Input: part model. Units: mm. Frame: model coordinates. A direction names the side the tool comes from. Round coordinates to 2 decimals unless told otherwise and drop trailing zeros. Loops run counter-clockwise (first coordinate to the right, second up) from the corner with the lowest first, then second, coordinate; pieces in that order, holes last. Notation, with made-up numbers: M -30.75,82 L -15.75,82 A24 cw -15.75,93 Z; hole C -25.5,57.25 d5. An arc over 180 degrees is marked long. Return JSON: item names as keys, results as strings. Group by question number.
1) Mould query, pull axis X, two halves, no side actions, for faces 1 (the face through (-29, 8, -32)), 2 (the face through (33, 8, 36)), 3 (the face through (7, 5, -1)). Classes: +X half, -X half, draft (parallel to the pull), parting line (faces both ways), or undercut.
2) Access query for faces 4 (the face through (28, 10, -38)), 5 (the face through (35, 2, 1)), 6 (the face through (29, 8, -32)), 7 (the face through (25, 8, -36)), 8 (the face through (4.75, 3, 0)). Directions: +Z, -Z, +X, -X, +Y, -Y. A direction counts if a zero-diameter tool reaches every point of the face in a straight line with its end or side. Return the directions, or none.
3) Contact query for flat-ended pins moving along their axis: P1, Ø2, axis at y = 7.5, z = -36, coming from the -X side; P2, Ø3, axis at x = 29, z = -36, coming from the -Y side; P3, Ø3, axis at y = 8.5, z = -38, coming from the +X side; P4, Ø4, axis at x = 21.5, z = -17.5, coming from the +Y side. Output: stop coordinate, or through.
4) Section A-A (z = 2). Output: boundary loops of the cut face in (x, y), plus the area to 4 significant figures.
5) Section B-B (y = 7). Output: boundary loops of the cut face in (x, z), plus the area to 3 significant figures.
6) Section C-C (z = 36). Output: boundary loops of the cut face in (x, y).
7) Material intervals for line 1 (X direction, y = 6.5, z = -36); line 2 (X direction, y = 3, z = 36); line 3 (X direction, y = 3.5, z = 2.5), sorted ascending. Write a range as from..to.
8) Section D-D (x = 29). Output: boundary loops of the cut face in (y, z).
from build123d import *

# Parameters (mm, degrees)
SKETCH_1_W          = 70
SKETCH_1_H          = 80
EXTRUDE_1_DEPTH     = 5
SKETCH_3_W          = 8
SKETCH_3_H          = 8
EXTRUDE_3_DEPTH     = 5
SKETCH_12_R         = 2
SKETCH_12_W         = 9.5
SKETCH_12_H         = 9.5
CUT_EXTRUDE_2_DEPTH = 10
FILLET_1_R          = 1


with BuildPart() as part:
    # 草圖1 → 填料-伸長1 (new body)
    with BuildSketch(Plane(origin=(0, 0, 0), x_dir=(1, 0, 0), z_dir=(0, 1, 0))):
        Rectangle(SKETCH_1_W, SKETCH_1_H)
    extrude(amount=EXTRUDE_1_DEPTH)

    # 草圖3 → 填料-伸長3 (add)
    with BuildSketch(Plane(origin=(0, 5, 0), x_dir=(1, 0, 0), z_dir=(0, 1, 0))):
        with Locations((-29, -36)):
            Rectangle(SKETCH_3_W, SKETCH_3_H)
        with Locations((-29, 36)):
            Rectangle(SKETCH_3_W, SKETCH_3_H)
        with Locations((29, -36)):
            Rectangle(SKETCH_3_W, SKETCH_3_H)
        with Locations((29, 36)):
            Rectangle(SKETCH_3_W, SKETCH_3_H)
    extrude(amount=EXTRUDE_3_DEPTH)

    # 草圖12 → 除料-伸長2 (cut)
    with BuildSketch(Plane(origin=(0, 10, 0), x_dir=(1, 0, 0), z_dir=(0, 1, 0))):
        with Locations(Location((-29, 36, 0), (0, 0, 270))):
            Circle(SKETCH_12_R)
        with Locations(Location((-29, -36, 0), (0, 0, 90))):
            Circle(SKETCH_12_R)
        with Locations(Location((29, -36, 0), (0, 0, 270))):
            Circle(SKETCH_12_R)
        with Locations(Location((29, 36, 0), (0, 0, 90))):
            Circle(SKETCH_12_R)
        Rectangle(SKETCH_12_W, SKETCH_12_H)
    extrude(amount=-CUT_EXTRUDE_2_DEPTH, mode=Mode.SUBTRACT)

    # 圓角1
    fillet_1_edges = [part.edges().sort_by_distance(p)[0] for p in [
        (-33, 5, 36),
        (-25, 5, 36),
        (-29, 5, 32),
        (-33, 5, -36),
        (-29, 5, -32),
        (-25, 5, -36),
        (33, 5, 36),
        (29, 5, 32),
        (25, 5, 36),
        (33, 5, -36),
        (25, 5, -36),
        (29, 5, -32),
    ]]
    fillet(fillet_1_edges, radius=FILLET_1_R)


solid = part.part
Returned:
{
 "1": {"face 1": "draft", "face 2": "+X half", "face 3": "undercut"},
 "2": {"face 4": "+Z, -Z, +X, -X, +Y", "face 5": "+Z, -Z, +X, +Y, -Y", "face 6": "+X, -X, +Y", "face 7": "+Z, -Z, +Y", "face 8": "+Y, -Y"},
 "3": {"P1": "stops at x = -33", "P2": "passes through", "P3": "stops at x = 33", "P4": "stops at y = 5"},
 "4": {"outline": "M -35,0 L -4.75,0 L -4.75,5 L -35,5 Z; M 4.75,0 L 35,0 L 35,5 L 4.75,5 Z", "area": "302.5 mm^2"},
 "5": {"outline": "M -33,-40 L -25,-40 L -25,-32 L -33,-32 Z; M -33,32 L -25,32 L -25,40 L -33,40 Z; M 25,-40 L 33,-40 L 33,-32 L 25,-32 Z; M 25,32 L 33,32 L 33,40 L 25,40 Z; hole C -29,-36 d4; hole C -29,36 d4; hole C 29,-36 d4; hole C 29,36 d4", "area": "206 mm^2"},
 "6": {"outline": "M -35,0 L -31,0 L -31,10 L -33,10 L -33,6 A1 cw -34,5 L -35,5 Z; M -27,0 L 27,0 L 27,10 L 25,10 L 25,6 A1 cw 24,5 L -24,5 A1 cw -25,6 L -25,10 L -27,10 Z; M 31,0 L 35,0 L 35,5 L 34,5 A1 cw 33,6 L 33,10 L 31,10 Z"},
 "7": {"line 1": "x = -33..-31, -27..-25, 25..27, 31..33", "line 2": "x = -35..-31, -27..27, 31..35", "line 3": "x = -35..-4.75, 4.75..35"},
 "8": {"outline": "M 0,-40 L 10,-40 L 10,-38 L 0,-38 Z; M 0,-34 L 10,-34 L 10,-32 L 6,-32 A1 cw 5,-31 L 5,31 A1 cw 6,32 L 10,32 L 10,34 L 0,34 Z; M 0,38 L 10,38 L 10,40 L 0,40 Z"}
}
